Read the model definition and answer for the solid it produces. Units are mm, in the model's axes. Face numbers are marked on the shaded views. A direction names the side the tool comes from. Round coordinates to 2 decimals unless told otherwise and drop trailing zeros. Write each loop counter-clockwise with the first axis right and the second up, starting at its lowest first coordinate (ties: lowest second). Pieces come first, ordered by that corner, then holes.
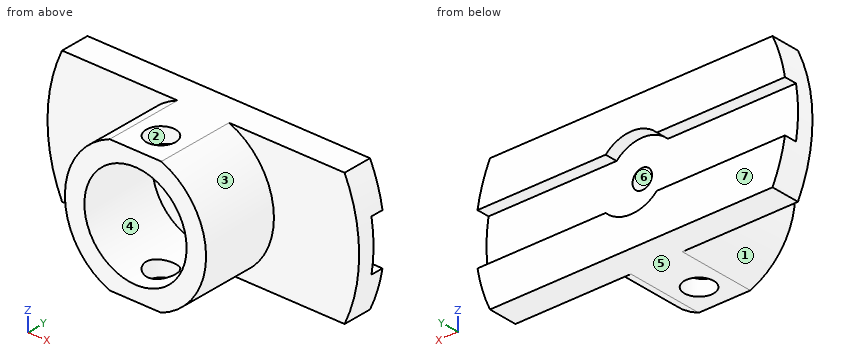
from build123d import *

# Parameters (mm, degrees)
SKETCH1_R               = 16
BOSS_EXTRUDE1_DEPTH     = 3
CUT_EXTRUDE1_START      = -1.3
CUT_EXTRUDE1_DEPTH      = 1.3
CUT_EXTRUDE3_DEPTH      = 2
CUT_EXTRUDE3_DEPTH_BACK = 2
SKETCH4_R               = 1
SKETCH5_R               = 7.25
SKETCH5_R_2             = 5.25
EXTRUDE_THIN1_DEPTH     = 8
CUT_EXTRUDE4_DEPTH      = 100
CUT_EXTRUDE4_DEPTH_BACK = 100
SKETCH6_W               = 10.574311585
SKETCH6_H               = 20.455042326
SKETCH6_W_2             = 9.477353479
SKETCH6_H_2             = 21.35841959
SKETCH7_R               = 1.5
CUT_EXTRUDE5_DEPTH      = 30
SKETCH8_R               = 3.7
CUT_EXTRUDE6_DEPTH      = 1.3


with BuildPart() as part:
    # Sketch1 → Boss-Extrude1 (new body)
    with BuildSketch(Plane(origin=(0, 0, 0), x_dir=(1, 0, 0), z_dir=(0, 1, 0))):
        with Locations(Location((0, 0, 0), (0, 0, 270))):
            Circle(SKETCH1_R)
    extrude(amount=BOSS_EXTRUDE1_DEPTH)

    # Sketch2 → Cut-Extrude1 (cut)
    with BuildSketch(Plane(origin=(0, 3, 0), x_dir=(1, 0, 0), z_dir=(0, 1, 0)).offset(CUT_EXTRUDE1_START)):
        with BuildLine():
            Line((-15.787336697, 2.6), (-2.343074903, 2.6))
            ThreePointArc((-2.343074903, 2.6), (0, 3.5), (2.343074903, 2.6))
            Line((2.343074903, 2.6), (15.787336697, 2.6))
            ThreePointArc((15.787336697, 2.6), (16, 0), (15.787336697, -2.6))
            Line((15.787336697, -2.6), (2.343074903, -2.6))
            ThreePointArc((2.343074903, -2.6), (0, -3.5), (-2.343074903, -2.6))
            Line((-2.343074903, -2.6), (-15.787336697, -2.6))
            ThreePointArc((-15.787336697, -2.6), (-16, 0), (-15.787336697, 2.6))
        make_face()
    extrude(amount=CUT_EXTRUDE1_DEPTH, mode=Mode.SUBTRACT)

    # Sketch4 → Cut-Extrude3 (cut, two sides: drawn at the far end of the back side and taken through both)
    with BuildSketch(Plane.XZ.offset(-0.3).offset(-CUT_EXTRUDE3_DEPTH_BACK)):
        with Locations(Location((0, 0, 0), (0, 0, 90))):
            Circle(SKETCH4_R)
    extrude(amount=CUT_EXTRUDE3_DEPTH + CUT_EXTRUDE3_DEPTH_BACK, mode=Mode.SUBTRACT)

    # Sketch5 → Extrude-Thin1 (add)
    with BuildSketch(Plane.XZ):
        Circle(SKETCH5_R)
        Circle(SKETCH5_R_2, mode=Mode.SUBTRACT)
    extrude(amount=EXTRUDE_THIN1_DEPTH)

    # Sketch6 → Cut-Extrude4 (cut, two sides: drawn at the far end of the back side and taken through both)
    with BuildSketch(Plane(origin=(0, 0, 0), x_dir=(0, 0, -1), z_dir=(1, 0, 0)).offset(-CUT_EXTRUDE4_DEPTH_BACK)):
        with Locations((-12.037155793, -3.839018001)):
            Rectangle(SKETCH6_W, SKETCH6_H)
        with Locations((11.48867674, -4.290706633)):
            Rectangle(SKETCH6_W_2, SKETCH6_H_2)
    extrude(amount=CUT_EXTRUDE4_DEPTH + CUT_EXTRUDE4_DEPTH_BACK, mode=Mode.SUBTRACT)

    # Sketch7 → Cut-Extrude5 (cut)
    with BuildSketch(Plane(origin=(0, 0, -6.75), x_dir=(-1, 0, 0), z_dir=(0, 0, -1))):
        with Locations(Location((0, -5, 0), (0, 0, 90))):
            Circle(SKETCH7_R)
    extrude(amount=-CUT_EXTRUDE5_DEPTH, mode=Mode.SUBTRACT)

    # Sketch8 → Cut-Extrude6 (cut)
    with BuildSketch(Plane(origin=(0, 3, 0), x_dir=(1, 0, 0), z_dir=(0, 1, 0))):
        Circle(SKETCH8_R)
    extrude(amount=-CUT_EXTRUDE6_DEPTH, mode=Mode.SUBTRACT)


solid = part.part
Q1. Section A-A (z = 0.5) is taken. Determine the outline of the cut face in (x, y), then the cut area to 3 significant figures.
Verdict:
outline: (-15.99, 0) - (-7.23, 0) - (-7.23, -8) - (-5.23, -8) - (-5.23, 0) - (-0.87, 0) - (-0.87, 1.7) - (-15.99, 1.7) - close; (0.87, 0) - (5.23, 0) - (5.23, -8) - (7.23, -8) - (7.23, 0) - (15.99, 0) - (15.99, 1.7) - (0.87, 1.7) - close
area: 83.5 mm2
Q2. Straight lines are drawn through the part: probe 1 along Y at (x, z) = (0, 6.2); probe 2 along X at (y, z) = (1.1, 0); probe 3 along Y at (x, z) = (9, -2.75). For each, find the intervals that lie inside material, in ascending order.
Verdict:
probe 1: y = -8 to -6.5, -3.5 to 3
probe 2: x = -16 to -1, 1 to 16
probe 3: y = 0 to 3
Q3. Section D-D (y = -1) is taken. Determine the outline of the cut face in (x, z).
Verdict:
outline: (-2.65, -6.75) - (2.65, -6.75) arc R7.25 ccw to (2.65, 6.75) - (-2.65, 6.75) arc R7.25 ccw to start; hole circle Ø10.5 at (0, 0)
Q4. Flat-ended cylindrical pins translate along their axes: pin 1 Ø4 at (y, z) = (-1.5, 2) entering from -X; pin 2 Ø5 at (y, z) = (-6, -4.5) entering from +X; pin 3 Ø1 at (y, z) = (-3, -1) entering from +X. Find the tip coordinate at first contact, or state that the pin passes through.
Verdict:
pin 1: stops at x = -15.99
pin 2: stops at x = 6.97
pin 3: stops at x = 7.23
Q5. Determine the mould class of the marked faces 5, 6 and 7 for opening direction Z: pulls with the +Z half, pulls with the -Z half, needs draft (parallel to the pull), parting line crosses it, or undercut.
Verdict:
face 5: pulls with the -Z half
face 6: undercut
face 7: needs draft
Q6. Section C-C (x = -10) is taken. Determine the outline of the cut face in (y, z), then the cut area to 3 significant figures.
Verdict:
outline: (0, -6.75) - (3, -6.75) - (3, -2.6) - (1.7, -2.6) - (1.7, 2.6) - (3, 2.6) - (3, 6.75) - (0, 6.75) - close
area: 33.7 mm2
Q7. Section B-B (y = -5) is taken. Determine the outline of the cut face in (x, z), then the cut area to 3 significant figures.
Verdict:
outline: (-2.65, -6.75) - (-1.5, -6.75) - (-1.5, -5.03) arc R5.25 cw to (-1.5, 5.03) - (-1.5, 6.75) - (-2.65, 6.75) arc R7.25 ccw to start; (1.5, -6.75) - (2.65, -6.75) arc R7.25 ccw to (2.65, 6.75) - (1.5, 6.75) - (1.5, 5.03) arc R5.25 cw to (1.5, -5.03) - close
area: 65.6 mm2
Q8. Which of the six approach directions +Z, -Z, +X, -X, +Y, -Y give full straight-line access (tool end or side, diameter ignored) to the marked faces 1, 2, 3 and 4?
Verdict:
face 1: -X, -Y
face 2: +Z, -Z
face 3: +X, -Y
face 4: -Y
